Part model, mm, in its own coordinate system. Face numbers are marked on the shaded views. A direction names the side the tool comes from. Coordinates: 2 decimals unless noted, no trailing zeros. Write each loop counter-clockwise with the first axis right and the second up, starting at its lowest first coordinate (ties: lowest second). Pieces come first, ordered by that corner, then holes. Notation, with made-up numbers: M 10,76.5 L 40,76.5 A18 cw 40,94.5 Z; hole C 32.5,-3 d11. An arc over 180 degrees is marked long. Use a Markdown table: item, result. Add a question column.
Q1. Pin check, flat tips, straight feed: pin 1 Ø1.4 at (x, z) = (4, 5) entering from +Y; pin 2 Ø1 at (y, z) = (1.5, 5) entering from -X. Stop position of each tip, or through.
Q2. Slice it at A-A on z = 5. Write the cut outline in (x, y), then the cut area to 3 significant figures.
Q3. Slice it at B-B on y = 1.5. Write the cut outline in (x, z), then the cut area to 3 significant figures.
Q4. Slice it at C-C on x = 3.25. Write the cut outline in (y, z), then the cut area to 3 significant figures.
Q5. Wall check: L1, parallel to X at y = 3.3, z = 1.75; L2, parallel to X at y = 1.2, z = 8; L3, parallel to Y at x = 2.75, z = 0.75. Give the ranges that are in metal, low to high. Write a range as from..to.
Q6. Tool access for the marked faces 1, 2 and 3: list every direction of +Z, -Z, +X, -X, +Y, -Y with a clear straight run to the whole face (end or side of a thin tool).
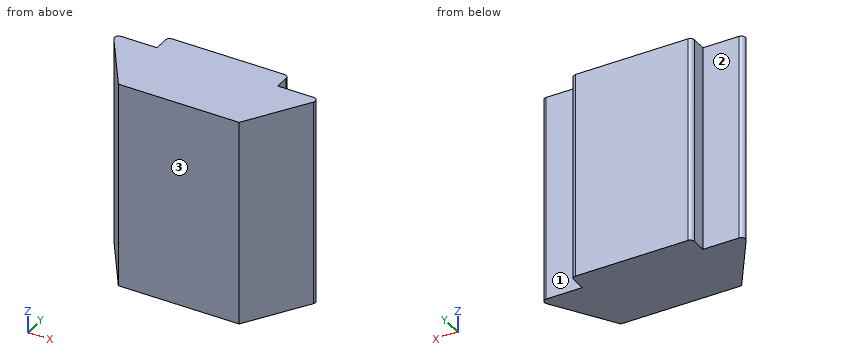
Autodesk Inventor part; units mm, degrees
ref_plane "YZ Plane" through (0, 0, 0) normal (1, 0, 0) x (0, 1, 0)
ref_plane "XZ Plane" through (0, 0, 0) normal (0, 1, 0) x (-1, 0, 0)
ref_plane "XY Plane" through (0, 0, 0) normal (0, 0, 1) x (1, 0, 0)
sketch "スケッチ1" plane through (0, 0, 0) normal (0, 0, 1) x (1, 0, 0)
  line L0 (0, 0) -> (2.9, 0)
  line L1 (2.9, 0) -> (5, 3.2)
  line L2 (5, 3.2) -> (0, 3.2)
  line L3 (0, 0) -> (0, 4)
  line L4 (0, 3.2) -> (2.9, 3.2)
  line L5 (2.9, 3.2) -> (2.9, 4.1)
  line L6 (2.9, 4.1) -> (0, 4.1)
  line L7 (0, 4.1) -> (0, 3.2)
  line L8 (0, 0) -> (-2.9, 0)
  line L9 (-2.9, 0) -> (-5, 3.2)
  line L10 (-5, 3.2) -> (0, 3.2)
  line L11 (-2.9, 3.2) -> (-2.9, 4.1)
  line L12 (-2.9, 4.1) -> (0, 4.1)
  dimension "d0" = 3.2
  dimension "d1" = 5
  dimension "d2" = 2.9
  dimension "d3" = 2.9
  dimension "d4" = 4.1
extrude "押し出し1" add sketch "スケッチ1" along normal blind 10
fillet "フィレット1" radius 0.2 2 edges at (5, 3.2, 5) (-5, 3.2, 5)
fillet "フィレット2" radius 0.2 2 edges at (-2.9, 4.1, 5) (2.9, 4.1, 5)
properties part number "framespacer1"
Recorded:
| question | item | result |
|---|---|---|
| 1 | pin 1 | y = 3.2 |
| 1 | pin 2 | x = -4.21 |
| 2 | outline | M -4.8,2.89 L -2.9,0 L 2.9,0 L 4.8,2.89 A0.2 ccw 4.63,3.2 L 2.9,3.2 L 2.9,3.9 A0.2 ccw 2.7,4.1 L -2.7,4.1 A0.2 ccw -2.9,3.9 L -2.9,3.2 L -4.63,3.2 A0.2 ccw Z |
| 2 | area | 30.4 mm² |
| 3 | outline | M -3.88,0 L 3.88,0 L 3.88,10 L -3.88,10 Z |
| 3 | area | 77.7 mm² |
| 4 | outline | M 0.53,0 L 3.2,0 L 3.2,10 L 0.53,10 Z |
| 4 | area | 26.7 mm² |
| 5 | L1 | -2.9..2.9 |
| 5 | L2 | -3.69..3.69 |
| 5 | L3 | 0..4.09 |
| 6 | face 1 | +Z, -Z, +X, +Y |
| 6 | face 2 | +Z, -Z, -X, +Y |
| 6 | face 3 | +Z, -Z, +X, -X, -Y |
